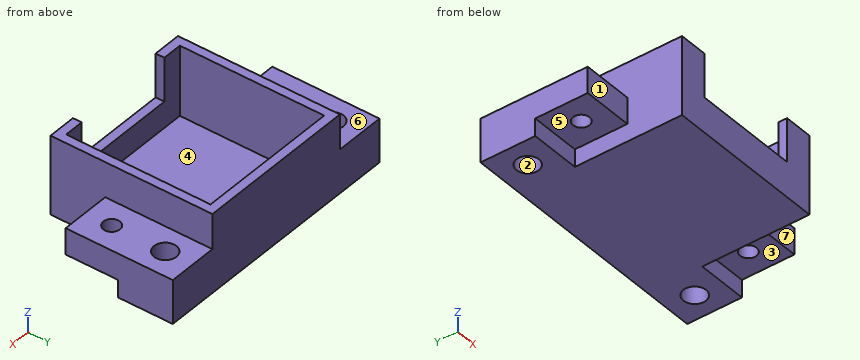
```python
from build123d import *

# Parameters (mm, degrees)
F0_W      = 29.36875
F0_H      = 29.36875
F0_W_2    = 26.19375
F0_H_2    = 26.19375
F1_DEPTH  = 14.2875
F2_W      = 26.19375
F2_H      = 26.19375
F3_DEPTH  = 1.5875
F7_W      = 19.05
F7_H      = 7.9375
F8_DEPTH  = 1.5875
F9_R      = 1.5
F10_DEPTH = 4.7625
F11_R     = 2.032
F12_DEPTH = 7.9375


with BuildPart() as f1:
    # F0 (on Top) → F1 (new body)
    with BuildSketch(Plane.XY):
        Rectangle(F0_W, F0_H)
        Rectangle(F0_W_2, F0_H_2, mode=Mode.SUBTRACT)
    extrude(amount=F1_DEPTH)

    # F2 (on face) → F3 (join)
    with BuildSketch(Plane(origin=(0, 0, 0), x_dir=(1, 0, 0), z_dir=(0, 0, -1))):
        Rectangle(F2_W, F2_H)
    extrude(amount=-F3_DEPTH)

    # F4: union 

    # F7 (on face) → F8 (cut, through all)
    with BuildSketch(Plane.XZ.offset(14.684375)):
        with Locations((0, 10.31875)):
            Rectangle(F7_W, F7_H)
    extrude(amount=-F8_DEPTH, mode=Mode.SUBTRACT)

    # F9 (on face) → F10 (join)
    with BuildSketch(Plane(origin=(0, 0, 3.175), x_dir=(1, 0, 0), z_dir=(0, 0, -1))):
        Polygon((23.8125, 4.7625), (19.2484375, 4.7625), (14.684375, 4.7625), (14.684375, -4.7625), (19.2484375, -4.7625), (23.8125, -4.7625), align=None)
        with Locations((19.2484375, 0)):
            Circle(F9_R, mode=Mode.SUBTRACT)
        Polygon((-19.2484375, -4.7625), (-14.684375, -4.7625), (-14.684375, 4.7625), (-19.2484375, 4.7625), (-23.8125, 4.7625), (-23.8125, -4.7625), align=None)
        with Locations((-19.2484375, 0)):
            Circle(F9_R, mode=Mode.SUBTRACT)
    extrude(amount=-F10_DEPTH)

    # F11 (on face) → F12 (join, through all)
    with BuildSketch(Plane(origin=(0, 0, 0), x_dir=(1, 0, 0), z_dir=(0, 0, -1))):
        Polygon((-23.8125, -14.684375), (-19.2484375, -14.684375), (-14.684375, -14.684375), (-14.684375, -4.7625), (-19.2484375, -4.7625), (-23.8125, -4.7625), align=None)
        with Locations((-19.2484375, -9.7234375)):
            Circle(F11_R, mode=Mode.SUBTRACT)
        Polygon((14.684375, -14.684375), (19.2484375, -14.684375), (23.8125, -14.684375), (23.8125, -4.7625), (19.2484375, -4.7625), (14.684375, -4.7625), align=None)
        with Locations((19.2484375, -9.7234375)):
            Circle(F11_R, mode=Mode.SUBTRACT)
    extrude(amount=-F12_DEPTH)


solid = f1.part
```
Input: part model. Units: mm. Frame: model coordinates. Face numbers are marked on the shaded views. A direction names the side the tool comes from. Give positions to 0.01 mm unless a question says otherwise; leave off trailing zeros. Write each loop counter-clockwise with the first axis right and the second up, starting at its lowest first coordinate (ties: lowest second). Pieces come first, ordered by that corner, then holes. Notation, with made-up numbers: (19, 34) - (71, 34) arc R25 ccw to (71, 71) - close; hole circle Ø8 at (-29, -28). An arc over 180 degrees is marked (long way). Write item = value, one per line. Start each with the question number.
1) Material intervals for L1, parallel to X at y = 0, z = 6.4; L2, parallel to X at y = 13, z = 8; L3, parallel to X at y = 8.25, z = 7.5, sorted ascending. Write a range as [from, to].
2) Cut plane C-C (z = 9.5). Return loops of the section in (x, y) (3 decimals).
3) Draft query along Y for the marked faces 1, 2 and 3. Return one class per face: pulls with the +Y half, pulls with the -Y half, needs draft (parallel to the pull), parting line crosses it, or undercut.
4) Cut plane D-D (y = -7.25). Return loops of the section in (x, z).
5) Cut plane B-B (x = -1). Return loops of the section in (y, z), and give its area (3 significant figures).
6) Cut plane A-A (y = 0). Return loops of the section in (x, z) (1 decimal), and give its area (3 significant figures).
7) Reachability of the marked faces 4, 5, 6 and 7 from +Z, -Z, +X, -X, +Y, -Y: full face, straight path, thin tool, end or side. Return the list, or none.
8) Pin query (flat end, axial travel): pin 1 (5 mm diameter, centred on y = -10.5, z = 12, fed in from -X); pin 2 (8 mm diameter, centred on x = -0.5, y = -1, fed in from +Z); pin 3 (8 mm diameter, centred on y = -10.5, z = 7.5, fed in from +X); pin 4 (2.5 mm diameter, centred on x = -19.25, y = 9.72, fed in from -Z). Return the tip coordinate at first contact, or that it passes through.
Answers follow:
q1.L1 = [-23.81, -20.75], [-17.75, -13.1], [13.1, 17.75], [20.75, 23.81]
q1.L2 = [-14.68, -13.1], [13.1, 14.68]
q1.L3 = [-23.81, -20.65], [-17.85, -13.1], [13.1, 17.85], [20.65, 23.81]
q2.outline = (-14.684, -14.684) - (-9.525, -14.684) - (-9.525, -13.097) - (-13.097, -13.097) - (-13.097, 13.097) - (13.097, 13.097) - (13.097, -13.097) - (9.525, -13.097) - (9.525, -14.684) - (14.684, -14.684) - (14.684, 14.684) - (-14.684, 14.684) - close
q3.face_1 = pulls with the -Y half
q3.face_2 = undercut
q3.face_3 = needs draft
q4.outline = (-14.68, 0) - (14.68, 0) - (14.68, 14.29) - (13.1, 14.29) - (13.1, 1.59) - (-13.1, 1.59) - (-13.1, 14.29) - (-14.68, 14.29) - close
q5.outline = (-14.68, 0) - (14.68, 0) - (14.68, 14.29) - (13.1, 14.29) - (13.1, 1.59) - (-13.1, 1.59) - (-13.1, 6.35) - (-14.68, 6.35) - close
q5.area = 74.3 mm^2
q6.outline = (-23.8, 3.2) - (-20.7, 3.2) - (-20.7, 7.9) - (-23.8, 7.9) - close; (-17.7, 3.2) - (-14.7, 3.2) - (-14.7, 0) - (14.7, 0) - (14.7, 3.2) - (17.7, 3.2) - (17.7, 7.9) - (14.7, 7.9) - (14.7, 14.3) - (13.1, 14.3) - (13.1, 1.6) - (-13.1, 1.6) - (-13.1, 14.3) - (-14.7, 14.3) - (-14.7, 7.9) - (-17.7, 7.9) - close; (20.7, 3.2) - (23.8, 3.2) - (23.8, 7.9) - (20.7, 7.9) - close
q6.area = 145 mm^2
q7.face_4 = +Z
q7.face_5 = -Z, -X, -Y
q7.face_6 = +Z, -X, +Y, -Y
q7.face_7 = +Z, -Z, +X, -Y
q8.pin_1 = -14.68
q8.pin_2 = 1.59
q8.pin_3 = 14.68
q8.pin_4 = through
